The listing builds one solid part. Answer for the finished solid, in the listing's coordinates (mm). A direction names the side the tool comes from. Round coordinates to 2 decimals unless told otherwise and drop trailing zeros. Order: outer loops, then holes, each group sorted by start corner. A loop starts at its lowest first (then second) coordinate and runs counter-clockwise, first axis right, second up. Notation, with made-up numbers: (55, 25.25) - (80, 25.25) arc R10 ccw to (80, 29.25) - close; hole circle Ø10 at (-39, 4). An arc over 180 degrees is marked (long way). Use CSV: the item, a comma, the result in double quotes. Start each with the question number.
Item 1: Determine the mould class of faces 1 (the flat face through (277.993, 65.501, -1076.121)), 2 (the flat face through (287, 10, -1033)), 3 (the flat face through (288.93, 75.52, -1078.3)) for opening direction X: +X half, -X half, draft (parallel to the pull), parting line (faces both ways), or undercut.
Item 2: Straight lines are drawn through the part: line 1 along X through (y, z) = (26.5, -1120); line 2 along X through (y, z) = (67, -1067); line 3 along Y through (x, z) = (-249, -1121.5). For each, find the intervals that lie inside material, in ascending order. Write a range as [from, to].
Item 3: For faces 4 (the flat face through (-288.4, 10, -1038.2)), 5 (the flat face through (-277.993, 65.501, -1076.121)), 6 (the cylindrical face through (3.299, 79.56, -899.994)), determine the directions among +Z, -Z, +X, -X, +Y, -Y from which every point of the face is accessible in a straight line to the end or side of a thin tool.
Item 4: Flat-ended cylindrical pins translate along their axes: P1, Ø6.5, axis at x = 310.54, z = -1120.3, coming from the +Y side; P2, Ø3.5, axis at x = 265.24, z = -951.26, coming from the -Y side; P3, Ø1.5, axis at y = 27.5, z = -1122.5, coming from the +X side; P4, Ø5, axis at x = 171.5, z = -1093, coming from the +Y side. Find the tip coordinate at first contact, or state that the pin passes through.
Item 5: Find section A-A, the plane y = 34.5. Give the vertices of the cut face in (x, z).
```python
from build123d import *

# Parameters (mm, degrees)
REVOLVE_1_ANGLE             = 15
REVOLVE_1_OTHER_WAY_ANGLE   = 15
EXTRUDE_1_REACH             = 1305.891
SKETCH_6_W                  = 350.000000001
SKETCH_6_H                  = 10
EXTRUDE_2_DEPTH             = 20
SKETCH_7_W                  = 350.000000001
SKETCH_7_H                  = 10
EXTRUDE_3_DEPTH             = 20
HOLE_WIZARD_M51_D           = 4.2
HOLE_WIZARD_M51_ON_FACE_2_D = 4.2
HOLE_WIZARD_M51_ON_FACE_3_D = 4.2
HOLE_WIZARD_M52_D           = 4.2


with BuildPart() as part:
    # Эскиз2 → Повернуть1 (revolve)
    with BuildSketch(Plane(origin=(0, 0, 0), x_dir=(0, 0, -1), z_dir=(1, 0, 0))):
        with BuildLine():
            Line((1250.000000001, 181.562500008), (1250.000000001, 171.562500008))
            add(Edge.make_bspline(
                [(900, 74.490000004), (1075.000000001, 115.125000006), (1250.000000001, 171.562500008)],
                knots=[0.083425123, 0.083425123, 0.083425123, 0.917676354, 0.917676354, 0.917676354], degree=2))
            Line((900, 74.490000004), (900, 84.490000004))
            add(Edge.make_bspline(
                [(900, 84.490000004), (1075.000000001, 125.125000006), (1250.000000001, 181.562500008)],
                knots=[0.083425123, 0.083425123, 0.083425123, 0.917676354, 0.917676354, 0.917676354], degree=2))
        make_face()
    revolve(axis=Axis((0, 605.286784652, 0), (0, -1, 0)), revolution_arc=REVOLVE_1_ANGLE)

    # Эскиз2 → Повернуть1 other way (revolve)
    with BuildSketch(Plane(origin=(0, 0, 0), x_dir=(0, 0, -1), z_dir=(1, 0, 0))):
        with BuildLine():
            Line((1250.000000001, 181.562500008), (1250.000000001, 171.562500008))
            add(Edge.make_bspline(
                [(900, 74.490000004), (1075.000000001, 115.125000006), (1250.000000001, 171.562500008)],
                knots=[0.083425123, 0.083425123, 0.083425123, 0.917676354, 0.917676354, 0.917676354], degree=2))
            Line((900, 74.490000004), (900, 84.490000004))
            add(Edge.make_bspline(
                [(900, 84.490000004), (1075.000000001, 125.125000006), (1250.000000001, 181.562500008)],
                knots=[0.083425123, 0.083425123, 0.083425123, 0.917676354, 0.917676354, 0.917676354], degree=2))
        make_face()
    revolve(axis=Axis((0, 605.286784652, 0), (0, 1, 0)), revolution_arc=REVOLVE_1_OTHER_WAY_ANGLE)

    # Эскиз5 → Бобышка-Вытянуть1 (add, up to next)
    with BuildSketch(Plane(origin=(0, 0, 0), x_dir=(1, 0, 0), z_dir=(0, 1, 0)), mode=Mode.PRIVATE) as extrude_1_sk1:
        Polygon((-323.523806378, 1207.407282862), (-232.937140592, 869.33324366), (-223.323059362, 872.090037092), (-313.819371083, 1209.826870333), align=None)
    extrude_1_tool1 = extrude(extrude_1_sk1.sketch, amount=EXTRUDE_1_REACH, mode=Mode.PRIVATE) - part.part
    # Эскиз5 → Бобышка-Вытянуть1 (add, up to next)
    with BuildSketch(Plane(origin=(0, 0, 0), x_dir=(1, 0, 0), z_dir=(0, 1, 0)), mode=Mode.PRIVATE) as extrude_1_sk2:
        Polygon((323.523806378, 1207.407282862), (232.937140592, 869.33324366), (223.323059362, 872.090037092), (313.819371083, 1209.826870333), align=None)
    extrude_1_tool2 = extrude(extrude_1_sk2.sketch, amount=EXTRUDE_1_REACH, mode=Mode.PRIVATE) - part.part
    add(extrude_1_tool1.solids().sort_by_distance((-273.401648, 0, -1039.664143))[0])
    add(extrude_1_tool2.solids().sort_by_distance((273.401648, 0, -1039.664143))[0])

    # Эскиз6 → Бобышка-Вытянуть2 (add)
    with BuildSketch(Plane(origin=(0, 0, 0), x_dir=(0.25881904510252135, 0, 0.9659258262890682), z_dir=(-0.9659258262890681, 0, 0.2588190451025213))):
        with Locations((-1075, 5)):
            Rectangle(SKETCH_6_W, SKETCH_6_H)
    extrude(amount=EXTRUDE_2_DEPTH)

    # Эскиз7 → Бобышка-Вытянуть3 (add)
    with BuildSketch(Plane(origin=(0, 0, 0), x_dir=(0.25881904510252124, 0, -0.9659258262890682), z_dir=(0.9659258262890682, 0, 0.25881904510252124))):
        with Locations((1075, 5)):
            Rectangle(SKETCH_7_W, SKETCH_7_H)
    extrude(amount=EXTRUDE_3_DEPTH)

    # Отверстие обработанное метчиком M51 (through all)
    with Locations(Plane(origin=(229.986727308, 161.264444267, -1162.865785876), x_dir=(0, -0.28736490905, 0.957821178011), z_dir=(-0.056742261531, 0.956277993991, 0.286901923948))):
        with Locations((0, 0)):
            Hole(HOLE_WIZARD_M51_D / 2)

    # Отверстие обработанное метчиком M51 on face 2 (through all)
    with Locations(Plane(origin=(-229.986727308, 161.264444267, -1162.865785876), x_dir=(0, -0.287364977278, 0.957821157542), z_dir=(0.056741999278, 0.95627798783, 0.286901996349))):
        with Locations((0, 0)):
            Hole(HOLE_WIZARD_M51_ON_FACE_2_D / 2)

    # Отверстие обработанное метчиком M51 on face 3 (through all)
    with Locations(Plane(origin=(0, 94.55738613, -942.359672798), x_dir=(0, -0.23624700812, 0.971693033398), z_dir=(0, 0.971693033398, 0.23624700812))):
        with Locations((-1e-09, 0)):
            Hole(HOLE_WIZARD_M51_ON_FACE_3_D / 2)

    # Отверстие обработанное метчиком M52 (through all)
    with Locations(Plane(origin=(0, 10, 0), x_dir=(1, 0, 0), z_dir=(0, 1, 0))):
        with Locations((-310.536398195, 1120.300582611), (-287.889731748, 1035.782072811), (-265.243065302, 951.26356301), (310.536398196, 1120.300582611), (287.889731751, 1035.78207281), (265.243065306, 951.263563009)):
            Hole(HOLE_WIZARD_M52_D / 2)


solid = part.part
```
Worked out:
1,face 1,"undercut"
1,face 2,"draft"
1,face 3,"+X half"
2,line 1,"x = [-300.1, -289.75], [289.75, 300.1]"
2,line 2,"x = [-285.9, -275.55], [275.55, 285.9]"
2,line 3,"y = [140.25, 150.25]"
3,face 4,"+Z, -X, +Y"
3,face 5,"-Z, -Y"
3,face 6,"+Z, +Y, -Y"
4,P1,"stops at y = 10"
4,P2,"passes through"
4,P3,"stops at x = 300.97"
4,P4,"stops at y = 138.62"
5,outline,"(-323.52, -1207.41) - (-313.82, -1209.83) - (-223.32, -872.09) - (-232.94, -869.33) - close; (223.32, -872.09) - (313.82, -1209.83) - (323.52, -1207.41) - (232.94, -869.33) - close"
